Could you check a few things on this model? Use its own coordinates, in mm. A direction names the side the tool comes from. Coordinates: 2 decimals unless noted, no trailing zeros. Loops run counter-clockwise (first coordinate to the right, second up) from the corner with the lowest first, then second, coordinate; pieces in that order, holes last. Notation, with made-up numbers: (48.5, 66.5) -> (89.5, 66.5) arc R16 cw to (89.5, 95.5) -> close; hole circle Ø11 at (-25.75, 11). An arc over 180 degrees is marked (long way). One line per question, with ' | ' between items. Start each with the question number.
(1) If I drill on line 1 along Y through (x, z) = (235, 3.7); line 2 along X through (y, z) = (11.25, 3.7); line 3 along X through (y, z) = (21.5, 6.5), over which ranges is the centre line in solid material (lowest first)?
(2) Suppose I cut it at B-B (z = 7.5). Please give me the cut outline in (x, y).
(3) Which directions (+Z, -Z, +X, -X, +Y, -Y) give clear straight access to the entire face, cutting with the end or side of a thin tool? Please do faces 1 (the face through (123, 23, 0)), 2 (the face through (235, 22, 4.8)).
(4) Suppose I cut it at A-A (y = 24). Please give me the cut outline in (x, z), plus the area to 3 significant figures.
(5) I'm going to push flat-ended pins straight in: pin 1 Ø2.5 at (y, z) = (12.5, 7) entering from +X; pin 2 Ø3.5 at (x, y) = (235, 11.25) entering from +Z. Where does each tip first touch, or does it pass through?
Autodesk Fusion 360 part; units mm, degrees
sketch "Sketch1" plane through (0, 0, 0) normal (0, 0, 1) x (1, 0, 0)
  line L0 (0, 0) -> (250, 0)
  line L1 (250, 0) -> (250, 45)
  line L2 (250, 45) -> (0, 45)
  line L3 (0, 45) -> (0, 0)
  dimension "d1" = 250
  dimension "d2" = 45
extrude "Extrude1" add sketch "Sketch1" along normal blind 9.5
extrude "Extrude2" add 1 faces at (83.3333, 30, 9.5) along direction (0, 0, 1) blind 0.1
sketch "Sketch2" plane through (0, 0, 9.6) normal (0, 0, 1) x (-1, 0, 0)
  line L0 (0, -45) -> (0, 0)
  line L1 (0, 0) -> (-250, 0)
  line L2 (-250, 0) -> (-250, -45)
  line L3 (-250, -45) -> (0, -45)
  line L4 (-250, -45) -> (-220, -45)
  line L5 (-220, -45) -> (-220, 0)
  line L6 (-220, 0) -> (-250, 0)
  line L7 (-250, 0) -> (-250, -45)
  dimension "d7" = 30
extrude "Extrude3" cut sketch "Sketch2" against normal blind 4.8 contours L1 L2 L3 L4 L5 L6 L7
sketch "Sketch3" plane through (0, 0, 4.8) normal (0, 0, 1) x (-1, 0, 0)
  line L0 (-250, 0) -> (-250, -45)
  line L1 (-250, -45) -> (-220, -45)
  line L2 (-220, -45) -> (-220, 0)
  line L3 (-220, 0) -> (-250, 0)
  circle A0 centre (-235, -33.75) radius 1.55
  circle A1 centre (-235, -11.25) radius 1.55
  dimension "d10" = 3.1
  dimension "d11" = 3.1
extrude "Extrude4" cut sketch "Sketch3" against normal blind 23 contours A0 | A1
equation "d8 = ( -9.6 / 2 ) * 1 mm"
Checks:
1) line 1: y = 0 to 9.7, 12.8 to 32.2, 35.3 to 45 | line 2: x = 0 to 233.45, 236.55 to 250 | line 3: x = 0 to 220
2) outline: (0, 0) -> (220, 0) -> (220, 45) -> (0, 45) -> close
3) face 1: -Z, +X, -X, +Y, -Y | face 2: +Z, +X, +Y, -Y
4) outline: (0, 0) -> (250, 0) -> (250, 4.8) -> (220, 4.8) -> (220, 9.6) -> (0, 9.6) -> close | area: 2,260 mm^2
5) pin 1: stops at x = 220 | pin 2: stops at z = 4.8
